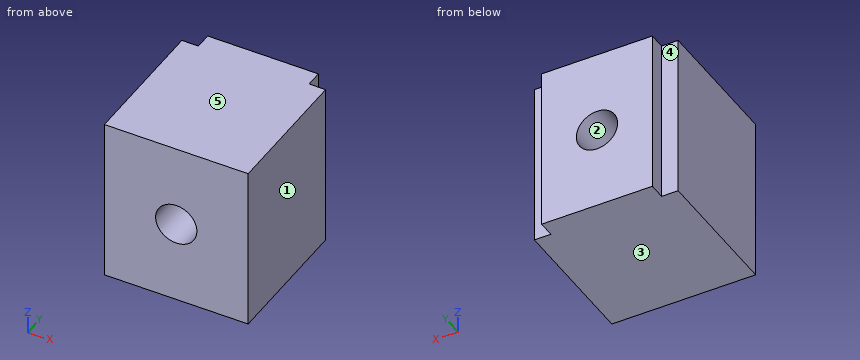
from build123d import *

# Parameters (mm, degrees)
SKETCH1_W           = 22.098
SKETCH1_H           = 25.4
SKETCH1_R           = 3.175
BOSS_EXTRUDE1_DEPTH = 23.749
SKETCH3_W           = 2.54
SKETCH3_H           = 25.4
CUT_EXTRUDE2_DEPTH  = 2.54


with BuildPart() as part:
    # Sketch1 → Boss-Extrude1 (new body)
    with BuildSketch(Plane(origin=(0, 0, 0), x_dir=(1, 0, 0), z_dir=(0, 1, 0))):
        Rectangle(SKETCH1_W, SKETCH1_H)
        with Locations(Location((0, 0, 0), (0, 0, 90))):
            Circle(SKETCH1_R, mode=Mode.SUBTRACT)
    extrude(amount=BOSS_EXTRUDE1_DEPTH)

    # Sketch3 → Cut-Extrude2 (cut)
    with BuildSketch(Plane(origin=(0, 23.749, 0), x_dir=(1, 0, 0), z_dir=(0, 1, 0))):
        with Locations((9.779, 0)):
            Rectangle(SKETCH3_W, SKETCH3_H)
        with Locations((-9.779, 0)):
            Rectangle(SKETCH3_W, SKETCH3_H)
    extrude(amount=-CUT_EXTRUDE2_DEPTH, mode=Mode.SUBTRACT)


solid = part.part
Work out the finished part from the listing and answer in its coordinate system (mm). Face numbers are marked on the shaded views. A direction names the side the tool comes from. Coordinates: 2 decimals unless noted, no trailing zeros. Order: outer loops, then holes, each group sorted by start corner. A loop starts at its lowest first (then second) coordinate and runs counter-clockwise, first axis right, second up. Notation, with made-up numbers: (35.5, -3) - (52.5, -3) arc R18 cw to (52.5, 15) - close; hole circle Ø11 at (36, 53). An arc over 180 degrees is marked (long way). Put each result on its own line as item: value. Start each with the question number.
1) For the marked faces 4 and 5, determine the directions among +Z, -Z, +X, -X, +Y, -Y from which every point of the face is accessible in a straight line to the end or side of a thin tool.
2) Find the intervals of material crossed by line 1 (X direction, y = 12.75, z = 0) (3 decimals); line 2 (X direction, y = 5, z = 0.5); line 3 (Z direction, x = 2, y = 18), in increasing order. Write a range as from..to.
3) Flat-ended cylindrical pins translate along their axes: pin 1 (1.3 mm diameter, centred on y = 23, z = 5, fed in from +X); pin 2 (1.3 mm diameter, centred on y = 22, z = 2, fed in from -X). Find the tip coordinate at first contact, or state that the pin passes through.
4) Find section A-A (z = 0). Give the vertices of the cut face in (x, y) (3 decimals), plus the area to 3 significant figures.
5) Find section C-C (y = 9). Give the vertices of the cut face in (x, z) (3 decimals).
6) For a pull along Z with two mould halves and no side action, classify the marked faces 1, 2 and 3 as released by +Z, released by -Z, zero draft, split by the parting line, or undercut.
7) Find section D-D (z = 10). Give the vertices of the cut face in (x, y).
8) Find section B-B (x = 0). Give the vertices of the cut face in (y, z) (3 decimals), plus the area to 3 significant figures.
Results list:
1. face 4: +Z, -Z, -X, +Y
1. face 5: +Z, +X, -X, +Y, -Y
2. line 1: x = -11.049..-3.175, 3.175..11.049
2. line 2: x = -11.05..-3.14, 3.14..11.05
2. line 3: z = -12.7..-2.47, 2.47..12.7
3. pin 1: stops at x = 8.51
3. pin 2: stops at x = -8.51
4. outline: (-11.049, 0) - (-3.175, 0) - (-3.175, 23.749) - (-8.509, 23.749) - (-8.509, 21.209) - (-11.049, 21.209) - close; (3.175, 0) - (11.049, 0) - (11.049, 21.209) - (8.509, 21.209) - (8.509, 23.749) - (3.175, 23.749) - close
4. area: 361 mm^2
5. outline: (-11.049, -12.7) - (11.049, -12.7) - (11.049, 12.7) - (-11.049, 12.7) - close; hole circle Ø6.35 at (0, 0)
6. face 1: zero draft
6. face 2: undercut
6. face 3: released by -Z
7. outline: (-11.05, 0) - (11.05, 0) - (11.05, 21.21) - (8.51, 21.21) - (8.51, 23.75) - (-8.51, 23.75) - (-8.51, 21.21) - (-11.05, 21.21) - close
8. outline: (0, -12.7) - (23.749, -12.7) - (23.749, -3.175) - (0, -3.175) - close; (0, 3.175) - (23.749, 3.175) - (23.749, 12.7) - (0, 12.7) - close
8. area: 452 mm^2
